Part model, mm, in its own coordinate system. Give positions to 0.01 mm unless a question says otherwise; leave off trailing zeros. Order: outer loops, then holes, each group sorted by start corner. A loop starts at its lowest first (then second) coordinate and runs counter-clockwise, first axis right, second up.
1. Mould opens along Z. For faces 1 (the cylindrical face through (27.9, 12, -2.7)), 2 (the cylindrical face through (27.7, -5.2, 16.5)) say: +Z half, -Z half, draft (parallel to the pull), parting line (faces both ways), or undercut.
2. Drop flat-ended pins along their axis: pin 1 Ø4 at (y, z) = (8, -33) entering from +X; pin 2 Ø10 at (y, z) = (-32.5, -16) entering from +X; pin 3 Ø3 at (y, z) = (9.5, -10.5) entering from +X. Give the stop position or say it passes through.
3. Probe line 1 (Y direction, x = 19, z = 0); line 2 (Z direction, x = 68.5, y = 5). List the from-to ranges inside material, lowest first.
4. Slice it at A-A on x = 49. List the corners of the cut face in (y, z).
5. Slice it at B-B on x = 61.5. List the corners of the cut face in (y, z), and give its area (3 significant figures).
from build123d import *

# Parameters (mm, degrees)
F2_R = 4.99999
F3_R = 15


# Not quite as in the source:
# - a fillet or chamfer is up to 0.001 mm smaller than in the source, because OpenCascade refuses the exact size


with BuildPart() as f1:
    # F0 (on Front) → F1 (revolve)
    with BuildSketch(Plane.XZ):
        Polygon((55, 17.3), (0, 17.3), (0, 12.3), (55, 12.3), (113.9615242271, 47.3), (106.9615242271, 47.3), align=None)
    revolve(axis=Axis((19.2044641059, 0, 0), (1, 0, 0)))

    # F2 (radius 5 in the source; OpenCascade refuses exactly that, so slightly less here)
    f2_edges = [f1.edges().sort_by_distance(p)[0] for p in [
        (0, 0, -17.3),
    ]]
    fillet(f2_edges, radius=F2_R)

    # F3
    f3_edges = [f1.edges().sort_by_distance(p)[0] for p in [
        (55, 0, -17.3),
    ]]
    fillet(f3_edges, radius=F3_R)


solid = f1.part
Data:
1. face 1: undercut
1. face 2: parting line
2. pin 1: stops at x = 94.85
2. pin 2: stops at x = 103.73
2. pin 3: stops at x = 60.66
3. line 1: y = -17.3 to -12.3, 12.3 to 17.3
3. line 2: z = -24.59 to -19.69, 19.69 to 24.59
4. outline: circle Ø34.6 at (0, 0); hole circle Ø24.6 at (0, 0)
5. outline: circle Ø42.11 at (0, 0); hole circle Ø32.32 at (0, 0)
5. area: 572 mm2
